Model file for the job. Use its own axes, mm. A direction names the side the tool comes from. Coordinates: 2 decimals unless noted, no trailing zeros. Order: outer loops, then holes, each group sorted by start corner. A loop starts at its lowest first (then second) coordinate and runs counter-clockwise, first axis right, second up. Notation, with made-up numbers: (88.25, 66) - (137.25, 66) arc R18 ccw to (137.25, 90) - close; hole circle Ø4 at (-19.5, 42). An arc over 180 degrees is marked (long way). Put each result on its own line as item: value. Start each with the question number.
```python
from build123d import *

# Parameters (mm, degrees)
SKETCH1_W           = 95.25
SKETCH1_H           = 177.8
BOSS_EXTRUDE1_DEPTH = 6.35
SKETCH2_W           = 12.7
SKETCH2_H           = 12.7
CUT_EXTRUDE1_DEPTH  = 7.35
LPATTERN1_COUNT     = 4
LPATTERN1_PITCH     = 25.4
SKETCH3_W           = 12.7
SKETCH3_H           = 6.35
CUT_EXTRUDE2_DEPTH  = 7.35
SKETCH5_W           = 6.35
SKETCH5_H           = 12.7
CUT_EXTRUDE4_DEPTH  = 7.35
LPATTERN2_COUNT     = 4
LPATTERN2_PITCH     = 25.4
SKETCH6_W           = 95.25
SKETCH6_H           = 38.1
CUT_EXTRUDE5_DEPTH  = 7.35
SKETCH7_W           = 12.7
SKETCH7_H           = 6.35
BOSS_EXTRUDE2_DEPTH = 6.35
LPATTERN3_COUNT     = 2
LPATTERN3_PITCH     = 25.4
LPATTERN3_COL_COUNT = 2
LPATTERN3_COL_PITCH = 25.4
LPATTERN4_COUNT     = 2
LPATTERN4_PITCH     = 76.2


with BuildPart() as part:
    # Sketch1 → Boss-Extrude1 (new body)
    with BuildSketch(Plane.XY):
        with Locations((47.625, 88.9)):
            Rectangle(SKETCH1_W, SKETCH1_H)
    extrude(amount=BOSS_EXTRUDE1_DEPTH)

    # Sketch2 → Cut-Extrude1 (cut, through all)
    with BuildSketch(Plane.XY.offset(6.35)):
        with Locations((6.35, 6.35)):
            Rectangle(SKETCH2_W, SKETCH2_H)
        with Locations((88.9, 6.35)):
            Rectangle(SKETCH2_W, SKETCH2_H)
    cut_extrude1 = extrude(amount=-CUT_EXTRUDE1_DEPTH, mode=Mode.SUBTRACT)

    # LPattern1: Cut-Extrude1 ×4
    with Locations(*[(0, i * LPATTERN1_PITCH, 0) for i in range(1, LPATTERN1_COUNT)]):
        add(cut_extrude1, mode=Mode.SUBTRACT)

    # Sketch3 → Cut-Extrude2 (cut, through all)
    with BuildSketch(Plane.XY.offset(6.35)):
        with Locations((34.925, 41.275)):
            Rectangle(SKETCH3_W, SKETCH3_H)
        with Locations((60.325, 41.275)):
            Rectangle(SKETCH3_W, SKETCH3_H)
    cut_extrude2 = extrude(amount=-CUT_EXTRUDE2_DEPTH, mode=Mode.SUBTRACT)

    # Sketch5 → Cut-Extrude4 (cut, through all)
    with BuildSketch(Plane.XY.offset(6.35)):
        with Locations((3.175, 107.95)):
            Rectangle(SKETCH5_W, SKETCH5_H)
        with Locations((92.075, 107.95)):
            Rectangle(SKETCH5_W, SKETCH5_H)
    cut_extrude4 = extrude(amount=-CUT_EXTRUDE4_DEPTH, mode=Mode.SUBTRACT)

    # LPattern2: Cut-Extrude4 ×4
    with Locations(*[(0, i * LPATTERN2_PITCH, 0) for i in range(1, LPATTERN2_COUNT)]):
        add(cut_extrude4, mode=Mode.SUBTRACT)

    # Sketch6 → Cut-Extrude5 (cut, through all)
    with BuildSketch(Plane.XY.offset(6.35)):
        with Locations((47.625, 158.75)):
            Rectangle(SKETCH6_W, SKETCH6_H)
    extrude(amount=-CUT_EXTRUDE5_DEPTH, mode=Mode.SUBTRACT)

    # Sketch7 → Boss-Extrude2 (add)
    with BuildSketch(Plane(origin=(0, 139.7, 0), x_dir=(1, 0, 0), z_dir=(0, 1, 0))):
        with Locations((47.625, -3.175)):
            Rectangle(SKETCH7_W, SKETCH7_H)
    boss_extrude2 = extrude(amount=BOSS_EXTRUDE2_DEPTH)

    # LPattern3: Boss-Extrude2 ×2
    with Locations(*[(i * LPATTERN3_PITCH, 0, 0) for i in range(1, LPATTERN3_COUNT)]):
        add(boss_extrude2)

    # LPattern3 col: Boss-Extrude2 ×2
    with Locations(*[(-i * LPATTERN3_COL_PITCH, 0, 0) for i in range(1, LPATTERN3_COL_COUNT)]):
        add(boss_extrude2)

    # LPattern4: Cut-Extrude2 ×2
    with Locations(*[(0, i * LPATTERN4_PITCH, 0) for i in range(1, LPATTERN4_COUNT)]):
        add(cut_extrude2, mode=Mode.SUBTRACT)


solid = part.part
```
Item 1: Slice it at D-D, the plane z = 5. Give the number of separate pieces and of enclosed holes in the cut face, plus the area to 3 significant figures.
Item 2: Slice it at B-B, the plane x = 9. Give the cut face in (y, z).
Item 3: 3-axis set-ups, long thin cutter, end or side, ignore diameter. For faces 4 (the face through (53.975, 41, 3)), 5 (the face through (92, 114.3, 3)), 6 (the face through (53.975, 143, 3)): which of +Z, -Z, +X, -X, +Y, -Y reach the whole face in a straight line?
Item 4: Flat gauge pins, fed straight in: pin 1 Ø3 at (x, z) = (7, 3.5) entering from -Y; pin 2 Ø3 at (y, z) = (106, 3) entering from +X; pin 3 Ø1.9 at (x, z) = (58, 3) entering from +Y. Where does each tip first touch, or does it go through?
Item 5: Wall check: line 1 along Y through (x, z) = (8.5, 4.25); line 2 along X through (y, z) = (39, 3.75) (3 decimals); line 3 along Y through (x, z) = (65, 3). Give the ranges that are in metal, low to high.
Item 6: Pull direction X, two halves, no side cores. Call faces 1 (the face through (3, 114.3, 3)), 2 (the face through (35, 114.3, 3)), 3 (the face through (0, 95, 3)): pulls with the +X half, pulls with the -X half, needs draft (parallel to the pull), parting line crosses it, or undercut.
Item 7: Slice it at A-A, the plane x = 56. Give the cut face in (y, z).
Item 8: Slice it at C-C, the plane y = 43. Give the cut face in (x, z) (3 decimals), plus the area to 3 significant figures.
Here are the results:
1. separate pieces: 1
1. enclosed holes: 4
1. area: 11,600 mm^2
2. outline: (12.7, 0) - (25.4, 0) - (25.4, 6.35) - (12.7, 6.35) - close; (38.1, 0) - (50.8, 0) - (50.8, 6.35) - (38.1, 6.35) - close; (63.5, 0) - (76.2, 0) - (76.2, 6.35) - (63.5, 6.35) - close; (88.9, 0) - (139.7, 0) - (139.7, 6.35) - (88.9, 6.35) - close
3. face 4: +Z, -Z
3. face 5: +Z, -Z, +X
3. face 6: +Z, -Z, +Y
4. pin 1: stops at y = 12.7
4. pin 2: stops at x = 88.9
4. pin 3: stops at y = 139.7
5. line 1: y = 12.7 to 25.4, 38.1 to 50.8, 63.5 to 76.2, 88.9 to 139.7
5. line 2: x = 0 to 28.575, 41.275 to 53.975, 66.675 to 95.25
5. line 3: y = 0 to 38.1, 44.45 to 114.3, 120.65 to 139.7
6. face 1: needs draft
6. face 2: undercut
6. face 3: pulls with the -X half
7. outline: (0, 0) - (38.1, 0) - (38.1, 6.35) - (0, 6.35) - close; (44.45, 0) - (114.3, 0) - (114.3, 6.35) - (44.45, 6.35) - close; (120.65, 0) - (139.7, 0) - (139.7, 6.35) - (120.65, 6.35) - close
8. outline: (0, 0) - (28.575, 0) - (28.575, 6.35) - (0, 6.35) - close; (41.275, 0) - (53.975, 0) - (53.975, 6.35) - (41.275, 6.35) - close; (66.675, 0) - (95.25, 0) - (95.25, 6.35) - (66.675, 6.35) - close
8. area: 444 mm^2
